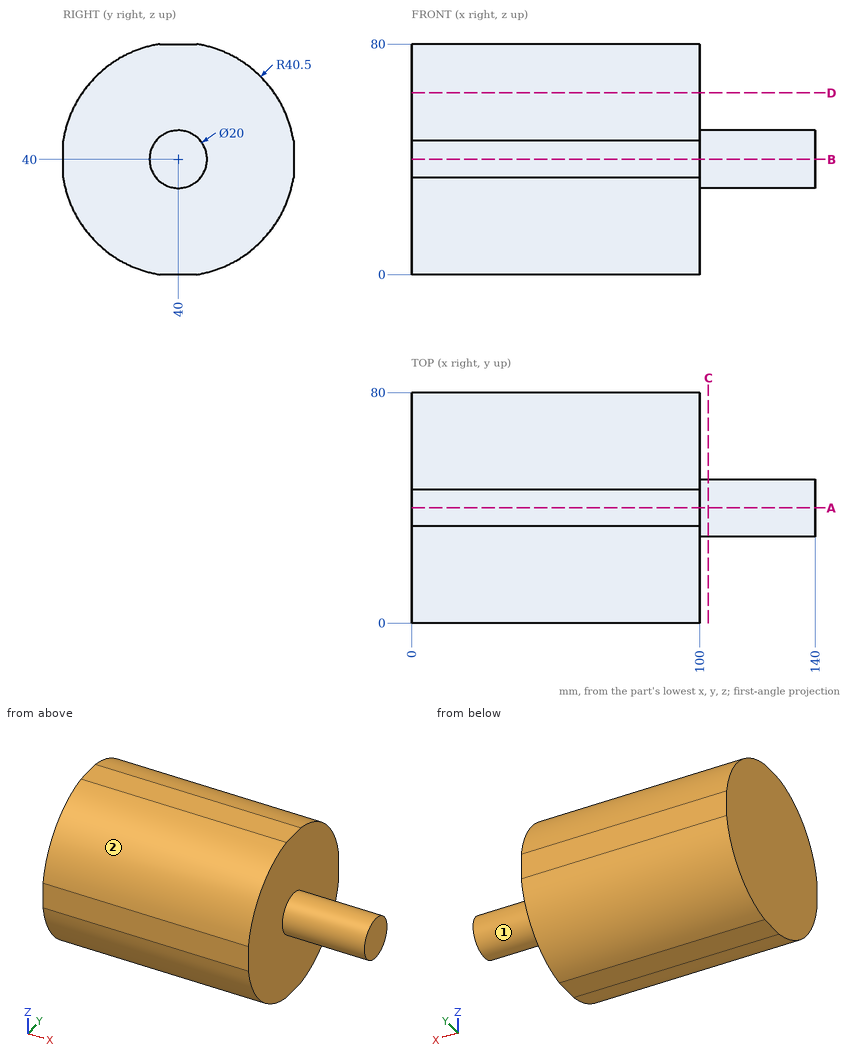
Drawing for the job (mm, zero at the part's lowest x, y, z). A direction names the side the tool comes from. Give positions to 0.01 mm unless a question says otherwise; leave off trailing zeros. Write each loop counter-clockwise with the first axis right and the second up, starting at its lowest first coordinate (ties: lowest second). Pieces come first, ordered by that corner, then holes. Notation, with made-up numbers: M -32,6.5 L 24,6.5 A18 ccw 24,38.5 Z; hole C 17.5,51 d1. An arc over 180 degrees is marked long. Return JSON: item names as keys, results as strings. Group by question number.
(1) Drill centre lines: L1, parallel to X at y = 60.5, z = 26; L2, parallel to Z at x = 61, y = 69.5; L3, parallel to Y at x = 93.5, z = 8. Where is each one in solid material? Low to high. Write a range as [from, to].
(2) Band-saw the part on D-D (z = 63). Give the cut face in (x, y), and give its area (3 significant figures).
(3) 3-axis set-ups, long thin cutter, end or side, ignore diameter. For the marked faces 1 and 2: which of +Z, -Z, +X, -X, +Y, -Y reach the whole face in a straight line?
(4) Band-saw the part on C-C (x = 103). Give the cut face in (y, z).
(5) Flat gauge pins, fed straight in: pin 1 Ø12 at (y, z) = (9.5, 8.5) entering from -X; pin 2 Ø1.5 at (x, z) = (68.5, 9.5) entering from +Y; pin 3 Ø8 at (x, y) = (39, 14.5) entering from -Z; pin 4 Ø1 at (x, y) = (34.5, 54.5) entering from -Z. Where does each tip first touch, or does it go through?
(6) Band-saw the part on A-A (y = 40). Give the cut face in (x, z), and give its area (3 significant figures).
Entries:
{
 "1": {"L1": "x = [0, 100]", "L2": "z = [12.25, 67.75]", "L3": "y = [15.18, 64.82]"},
 "2": {"outline": "M 0,6.66 L 100,6.66 L 100,73.34 L 0,73.34 Z", "area": "6,670 mm^2"},
 "3": {"face 1": "+X", "face 2": "+Z, +X, -X, -Y"},
 "4": {"outline": "C 40,40 d20"},
 "5": {"pin 1": "stops at x = 0", "pin 2": "stops at y = 67.48", "pin 3": "stops at z = 5.68", "pin 4": "stops at z = 2"},
 "6": {"outline": "M 0,0 L 100,0 L 100,30 L 140,30 L 140,50 L 100,50 L 100,80 L 0,80 Z", "area": "8,800 mm^2"}
}
